from build123d import *

# Parameters (mm, degrees)
BASE_EXTRUDE_THIN_DEPTH = 12.7
SKETCH2_R               = 3.175
CUT_EXTRUDE1_DEPTH      = 104.262871396
SKETCH3_R               = 1.587498625
CUT_EXTRUDE2_DEPTH      = 105.597511486
SKETCH4_R               = 1.587498625
CUT_EXTRUDE3_DEPTH      = 105.597511486


with BuildPart() as part:
    # Sketch1 → Base-Extrude-Thin (new, symmetric)
    with BuildSketch(Plane.XY):
        Polygon((53.34, 87.503), (53.34, 74.803), (0, 74.803), (0, -74.803), (53.34, -74.803), (53.34, -87.503), (55.88, -87.503), (55.88, -72.263), (2.54, -72.263), (2.54, 72.263), (55.88, 72.263), (55.88, 87.503), align=None)
    extrude(amount=BASE_EXTRUDE_THIN_DEPTH, both=True)

    # Sketch2 → Cut-Extrude1 (cut, through all)
    with BuildSketch(Plane(origin=(2.54, 0, 0), x_dir=(0, 0, -1), z_dir=(1, 0, 0))):
        with Locations(Location((0, 0, 0), (0, 0, 90))):
            Circle(SKETCH2_R)
    extrude(amount=-CUT_EXTRUDE1_DEPTH, mode=Mode.SUBTRACT)

    # Sketch3 → Cut-Extrude2 (cut, through all)
    with BuildSketch(Plane.ZY):
        with Locations(Location((0, 23.9776, 0), (0, 0, 270))):
            Circle(SKETCH3_R)
    extrude(amount=-CUT_EXTRUDE2_DEPTH, mode=Mode.SUBTRACT)

    # Sketch4 → Cut-Extrude3 (cut, through all)
    with BuildSketch(Plane.ZY):
        with Locations(Location((0, -23.9776, 0), (0, 0, 270))):
            Circle(SKETCH4_R)
    extrude(amount=-CUT_EXTRUDE3_DEPTH, mode=Mode.SUBTRACT)


solid = part.part
The listing builds one solid part. Answer for the finished solid, in the listing's coordinates (mm). A direction names the side the tool comes from. Give positions to 0.01 mm unless a question says otherwise; leave off trailing zeros. Order: outer loops, then holes, each group sorted by start corner. A loop starts at its lowest first (then second) coordinate and runs counter-clockwise, first axis right, second up. Notation, with made-up numbers: (-16, -27.75) - (15, -27.75) arc R17 ccw to (15, -9.75) - close; hole circle Ø4 at (42, -34.5). An arc over 180 degrees is marked (long way). Use one line per item in the form item = value.
1) Find section D-D on z = 9.5. Determine the outline of the cut face in (x, y).
Verdict:
outline = (0, -74.8) - (53.34, -74.8) - (53.34, -87.5) - (55.88, -87.5) - (55.88, -72.26) - (2.54, -72.26) - (2.54, 72.26) - (55.88, 72.26) - (55.88, 87.5) - (53.34, 87.5) - (53.34, 74.8) - (0, 74.8) - close
2) Consider probe 1 along Z at (x, y) = (1.9, 0) (3 decimals); probe 2 along Y at (x, z) = (34.5, -8.75); probe 3 along X at (y, z) = (50, -2). Determine where each line is inside the solid, lowest interval first. Write a range as [from, to].
Verdict:
probe_1 = [-12.7, -3.175], [3.175, 12.7]
probe_2 = [-74.8, -72.26], [72.26, 74.8]
probe_3 = [0, 2.54]
3) Find section A-A on z = 0. Determine the outline of the cut face in (x, y) (3 decimals), and give its area (3 significant figures).
Verdict:
outline = (0, -74.803) - (53.34, -74.803) - (53.34, -87.503) - (55.88, -87.503) - (55.88, -72.263) - (2.54, -72.263) - (2.54, -25.565) - (0, -25.565) - close; (0, -22.39) - (2.54, -22.39) - (2.54, -3.175) - (0, -3.175) - close; (0, 3.175) - (2.54, 3.175) - (2.54, 22.39) - (0, 22.39) - close; (0, 25.565) - (2.54, 25.565) - (2.54, 72.263) - (55.88, 72.263) - (55.88, 87.503) - (53.34, 87.503) - (53.34, 74.803) - (0, 74.803) - close
area = 683 mm^2
4) Find section B-B on y = 0. Determine the outline of the cut face in (x, z) (3 decimals).
Verdict:
outline = (0, -12.7) - (2.54, -12.7) - (2.54, -3.175) - (0, -3.175) - close; (0, 3.175) - (2.54, 3.175) - (2.54, 12.7) - (0, 12.7) - close
5) Each of these flat-tipped pins is pushed along its axis until it touches: pin 1 (7.5 mm diameter, centred on x = 14, z = 0.5, fed in from +Y); pin 2 (8 mm diameter, centred on x = 6.5, y = 40, fed in from -Z); pin 3 (4 mm diameter, centred on y = 83.5, z = 3.5, fed in from -X); pin 4 (2.5 mm diameter, centred on y = 23.98, z = 0, fed in from +X). Where does it stop, or does it pass through?
Verdict:
pin_1 = 74.8
pin_2 = -12.7
pin_3 = 53.34
pin_4 = through
6) The mould has two halves that part along Z. Classify faces 4 (the cylindrical face through (1.252, 25.564, 0.07)), 5 (the flat face through (26, -74.803, 0)), 6 (the flat face through (1, 0, -12.7)), 7 (the flat face through (1, 0, 12.7)): released by +Z, released by -Z, zero draft, split by the parting line, or undercut.
Verdict:
face_4 = undercut
face_5 = zero draft
face_6 = released by -Z
face_7 = released by +Z
7) For faces 1 (the flat face through (27, 74.803, 0)), 2 (the flat face through (53.34, -81, 0)), 3 (the flat face through (29, 72.263, 0)), determine the directions among +Z, -Z, +X, -X, +Y, -Y from which every point of the face is accessible in a straight line to the end or side of a thin tool.
Verdict:
face_1 = +Z, -Z, -X, +Y
face_2 = +Z, -Z, -X, -Y
face_3 = +Z, -Z, +X
8) Find section C-C on x = 15.5. Determine the outline of the cut face in (y, z).
Verdict:
outline = (-74.8, -12.7) - (-72.26, -12.7) - (-72.26, 12.7) - (-74.8, 12.7) - close; (72.26, -12.7) - (74.8, -12.7) - (74.8, 12.7) - (72.26, 12.7) - close
